Build history of the part. All positions in model axes, mm. A direction names the side the tool comes from. Coordinates: 2 decimals unless noted, no trailing zeros. One line per item, written item: value.
from build123d import *

# Parameters (mm, degrees)
SKETCH1_W           = 15
SKETCH1_H           = 15
SKETCH1_R           = 1.25
BOSS_EXTRUDE1_DEPTH = 45
FILLET1_R           = 0.25
CUT_EXTRUDE1_DEPTH  = 91.622844802
CUT_EXTRUDE3_DEPTH  = 91.622844802
FILLET3_R           = 0.5
FILLET4_R           = 0.5
FILLET5_R           = 3
FILLET6_R           = 0.2
CUT_EXTRUDE4_DEPTH  = 91.622844802
FILLET8_R           = 0.5
SKETCH6_W           = 5.1529354
SKETCH6_H           = 1.651
SKETCH6_W_2         = 1.651
SKETCH6_H_2         = 5.1529354
CUT_EXTRUDE5_DEPTH  = 91.622844802
FILLET10_R          = 0.2


with BuildPart() as part:
    # Sketch1 → Boss-Extrude1 (new, symmetric)
    with BuildSketch(Plane.XY):
        Rectangle(SKETCH1_W, SKETCH1_H)
        Circle(SKETCH1_R, mode=Mode.SUBTRACT)
    extrude(amount=BOSS_EXTRUDE1_DEPTH, both=True)

    # Fillet1
    fillet1_edges = [part.edges().sort_by_distance(p)[0] for p in [
        (7.5, -7.5, 0),
        (-7.5, -7.5, 0),
        (-7.5, 7.5, 0),
        (7.5, 7.5, 0),
    ]]
    fillet(fillet1_edges, radius=FILLET1_R)

    # Sketch2 → Cut-Extrude1 (cut, through all)
    with BuildSketch(Plane.XY.offset(45)):
        Polygon((-7.5, 1.6), (-6.1, 1.6), (-6.1, 2.9), (-3.4, 2.9), (-3.4, -2.9), (-6.1, -2.9), (-6.1, -1.6), (-7.5, -1.6), align=None)
        Polygon((2.9, 6.1), (1.6, 6.1), (1.6, 7.5), (-1.6, 7.5), (-1.6, 6.1), (-2.9, 6.1), (-2.9, 3.4), (2.9, 3.4), align=None)
        Polygon((-1.6, -7.5), (-1.6, -6.1), (-2.9, -6.1), (-2.9, -3.4), (2.9, -3.4), (2.9, -6.1), (1.6, -6.1), (1.6, -7.5), align=None)
        Polygon((6.1, -2.9), (6.1, -1.6), (7.5, -1.6), (7.5, 1.6), (6.1, 1.6), (6.1, 2.9), (3.4, 2.9), (3.4, -2.9), align=None)
    extrude(amount=-CUT_EXTRUDE1_DEPTH, mode=Mode.SUBTRACT)

    # Sketch4 → Cut-Extrude3 (cut, through all)
    with BuildSketch(Plane.XY.offset(45)):
        Polygon((-3.4, 2.9), (-2.75, 0), (-3.4, -2.9), align=None)
        Polygon((-2.9, 3.4), (0, 2.75), (2.9, 3.4), align=None)
        Polygon((3.4, 2.9), (2.75, 0), (3.4, -2.9), align=None)
        Polygon((-2.9, -3.4), (0, -2.75), (2.9, -3.4), align=None)
    extrude(amount=-CUT_EXTRUDE3_DEPTH, mode=Mode.SUBTRACT)

    # Fillet3
    fillet3_edges = [part.edges().sort_by_distance(p)[0] for p in [
        (1.6, -7.5, 0),
        (-1.6, -7.5, 0),
        (-1.6, -6.1, 0),
        (1.6, -6.1, 0),
        (6.1, 1.6, 0),
        (7.5, 1.6, 0),
        (7.5, -1.6, 0),
        (6.1, -1.6, 0),
        (-7.5, -1.6, 0),
        (-7.5, 1.6, 0),
        (-6.1, 1.6, 0),
        (-6.1, -1.6, 0),
        (-1.6, 6.1, 0),
        (-1.6, 7.5, 0),
        (1.6, 7.5, 0),
        (1.6, 6.1, 0),
    ]]
    fillet(fillet3_edges, radius=FILLET3_R)

    # Fillet4
    fillet4_edges = [part.edges().sort_by_distance(p)[0] for p in [
        (-2.9, -3.4, 0),
        (2.9, -3.4, 0),
        (3.4, -2.9, 0),
        (3.4, 2.9, 0),
        (-3.4, 2.9, 0),
        (-3.4, -2.9, 0),
        (2.9, 3.4, 0),
        (-2.9, 3.4, 0),
    ]]
    fillet(fillet4_edges, radius=FILLET4_R)

    # Fillet5
    fillet5_edges = [part.edges().sort_by_distance(p)[0] for p in [
        (-2.75, 0, 0),
        (0, 2.75, 0),
        (2.75, 0, 0),
        (0, -2.75, 0),
    ]]
    fillet(fillet5_edges, radius=FILLET5_R)

    # Fillet6
    fillet6_edges = [part.edges().sort_by_distance(p)[0] for p in [
        (-2.9, -6.1, 0),
        (2.9, -6.1, 0),
        (6.1, -2.9, 0),
        (6.1, 2.9, 0),
        (-6.1, 2.9, 0),
        (-6.1, -2.9, 0),
        (2.9, 6.1, 0),
        (-2.9, 6.1, 0),
    ]]
    fillet(fillet6_edges, radius=FILLET6_R)

    # Sketch5 → Cut-Extrude4 (cut, through all)
    with BuildSketch(Plane.XY.offset(45)):
        Polygon((-7.5, 6.439339828), (-5.460660172, 4.4), (-7.5, 4.4), align=None)
        Polygon((-6.439339828, 7.5), (-4.4, 5.460660172), (-4.4, 7.5), align=None)
        Polygon((4.4, 7.5), (6.439339828, 7.5), (4.4, 5.460660172), align=None)
        Polygon((7.5, 6.439339828), (7.5, 4.4), (5.460660172, 4.4), align=None)
        Polygon((7.5, -6.439339828), (5.460660172, -4.4), (7.5, -4.4), align=None)
        Polygon((6.439339828, -7.5), (4.4, -5.460660172), (4.4, -7.5), align=None)
        Polygon((-4.4, -7.5), (-6.439339828, -7.5), (-4.4, -5.460660172), align=None)
        Polygon((-7.5, -6.439339828), (-7.5, -4.4), (-5.460660172, -4.4), align=None)
    extrude(amount=-CUT_EXTRUDE4_DEPTH, mode=Mode.SUBTRACT)

    # Fillet8
    fillet8_edges = [part.edges().sort_by_distance(p)[0] for p in [
        (-7.5, 4.4, 0),
        (-7.5, 6.439339828, 0),
        (-5.460660172, 4.4, 0),
        (7.5, -4.4, 0),
        (7.5, -6.439339828, 0),
        (5.460660172, -4.4, 0),
        (5.460660172, 4.4, 0),
        (7.5, 6.439339828, 0),
        (7.5, 4.4, 0),
        (-4.4, 7.5, 0),
        (-4.4, 5.460660172, 0),
        (-6.439339828, 7.5, 0),
        (-5.460660172, -4.4, 0),
        (-7.5, -6.439339828, 0),
        (-7.5, -4.4, 0),
        (4.4, 5.460660172, 0),
        (4.4, 7.5, 0),
        (6.439339828, 7.5, 0),
        (6.439339828, -7.5, 0),
        (4.4, -7.5, 0),
        (4.4, -5.460660172, 0),
        (-6.439339828, -7.5, 0),
        (-4.4, -5.460660172, 0),
        (-4.4, -7.5, 0),
    ]]
    fillet(fillet8_edges, radius=FILLET8_R)

    # Sketch6 → Cut-Extrude5 (cut, through all)
    with BuildSketch(Plane.XY.offset(45)):
        with Locations((4.9235323, 0)):
            Rectangle(SKETCH6_W, SKETCH6_H)
        with Locations((0, -4.9235323)):
            Rectangle(SKETCH6_W_2, SKETCH6_H_2)
        with Locations((-4.9235323, 0)):
            Rectangle(SKETCH6_W, SKETCH6_H)
        with Locations((0, 4.9235323)):
            Rectangle(SKETCH6_W_2, SKETCH6_H_2)
    extrude(amount=-CUT_EXTRUDE5_DEPTH, mode=Mode.SUBTRACT)

    # Fillet10
    fillet10_edges = [part.edges().sort_by_distance(p)[0] for p in [
        (0.8255, -2.935025862, 0),
        (-0.8255, -2.935025862, 0),
        (0.8255, -2.3470646, 0),
        (-0.8255, -2.3470646, 0),
        (2.935025862, 0.8255, 0),
        (2.935025862, -0.8255, 0),
        (2.3470646, 0.8255, 0),
        (2.3470646, -0.8255, 0),
        (-2.935025862, -0.8255, 0),
        (-2.935025862, 0.8255, 0),
        (-2.3470646, -0.8255, 0),
        (-2.3470646, 0.8255, 0),
        (-0.8255, 2.935025862, 0),
        (0.8255, 2.935025862, 0),
        (-0.8255, 2.3470646, 0),
        (0.8255, 2.3470646, 0),
    ]]
    fillet(fillet10_edges, radius=FILLET10_R)


solid = part.part
1. 3-axis set-ups, long thin cutter, end or side, ignore diameter. For faces 5 (the face through (7.5, -3, 1)), 6 (the face through (-5, -2.9, 1)): which of +Z, -Z, +X, -X, +Y, -Y reach the whole face in a straight line?
Values found:
face 5: +Z, -Z, +X, +Y, -Y
face 6: +Z, -Z
2. Two-plate mould, pull along X, no slides. Class faces 1 (the face through (1.735, -3.139, 0.63)), 2 (the face through (3, -7.5, 1)), 3 (the face through (-1.756, 3.144, 0.63)), 4 (the face through (7.5, 3, 1)): pulls with the +X half, pulls with the -X half, needs draft (parallel to the pull), parting line crosses it, or undercut.
Values found:
face 1: undercut
face 2: needs draft
face 3: undercut
face 4: pulls with the +X half
3. Probe line 1 along X through (y, z) = (2.5, -37); line 2 along Y through (x, z) = (0, 0); line 3 along X through (y, z) = (-2.25, 21). List the from-to ranges inside material, lowest first.
Values found:
line 1: x = -7.5 to -6.1, -3.31 to -0.82, 0.82 to 3.31, 6.1 to 7.5
line 2: y = -2.35 to -1.25, 1.25 to 2.35
line 3: x = -7.5 to -6.1, -3.25 to 3.25, 6.1 to 7.5
4. Flat gauge pins, fed straight in: P1, Ø2, axis at y = -1, z = 16, coming from the -X side; P2, Ø1.4, axis at y = 0, z = -15, coming from the -X side; P3, Ø0.6, axis at y = 5, z = -17.5, coming from the +X side. Where does each tip first touch, or does it go through?
Values found:
P1: stops at x = -7.49
P2: stops at x = -2.36
P3: stops at x = 6.36
